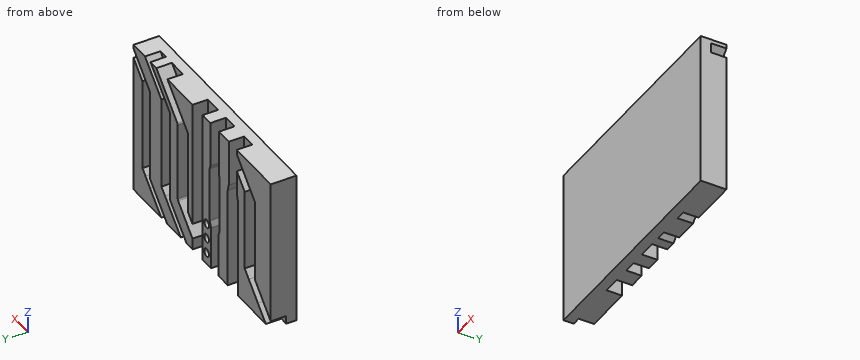
```python
from build123d import *

# Parameters (mm, degrees)
SKETCH1_W           = 292.1
SKETCH1_H           = 190.5
BOSS_EXTRUDE1_DEPTH = 31.75
CUT_EXTRUDE1_DEPTH  = 19.05
FILLET1_R           = 3.175
SKETCH8_R           = 5.08
CUT_EXTRUDE2_DEPTH  = 12.7
CUT_EXTRUDE3_DEPTH  = 19.05
CUT_EXTRUDE4_START  = -19.05
CUT_EXTRUDE4_DEPTH  = 19.05


with BuildPart() as part:
    # Sketch1 → Boss-Extrude1 (new body)
    with BuildSketch(Plane(origin=(0, 0, 0), x_dir=(1, 0, 0), z_dir=(0, 1, 0))):
        Rectangle(SKETCH1_W, SKETCH1_H)
    extrude(amount=BOSS_EXTRUDE1_DEPTH)

    # Sketch5 → Cut-Extrude1 (cut)
    with BuildSketch(Plane(origin=(0, 31.75, 0), x_dir=(1, 0, 0), z_dir=(0, 1, 0))):
        Polygon((-54.537973011, 56.645897063), (-54.537973011, 45.282587268), (-54.537973011, -9.143020761), (-54.537973011, -29.727810076), (-56.751368127, -37.988313106), (-56.751368127, -113.256317169), (-73.902361837, -113.256317169), (-73.902361837, -37.988313106), (-76.115756953, -29.727810076), (-76.115756953, -11.930912732), (-76.115756953, -9.143020761), (-76.115756953, 45.282587268), (-76.115756953, 56.645897063), (-76.115756953, 64.900897063), (-76.115756953, 123.938542293), (-54.537973011, 123.938542293), (-54.537973011, 64.900897063), align=None)
        Polygon((-35.869641097, -54.76875), (-35.869641097, -113.256317169), (-17.739641097, -113.256317169), (-17.739641097, -54.76875), (-17.739641097, -38.54651566), (-16.168929869, -34.231022029), (-16.168929869, 34.231022029), (-19.014641097, 42.04954937), (-19.014641097, 54.76875), (-19.014641097, 123.938542293), (-34.594641097, 123.938542293), (-34.594641097, 54.76875), (-34.594641097, 42.04954937), (-37.440352325, 34.231022029), (-37.440352325, -34.231022029), (-35.869641097, -38.54651566), align=None)
        Polygon((68.007088005, -12.827), (68.007088005, -53.93599914), (75.733185186, -61.662096321), (85.826970956, -71.755882091), (120.911645373, -106.060842413), (128.794129656, -102.532519884), (91.922231409, -65.660621637), (86.625610633, -60.36400086), (86.625610633, -12.827), (86.625610633, 12.827), (86.625610633, 54.107702226), (78.899513451, 61.662096321), (69.164333129, 71.397276643), (30.279619459, 110.281990313), (23.687738087, 104.683350778), (63.069072676, 65.302016189), (68.007088005, 60.36400086), (68.007088005, 12.827), align=None)
        Polygon((20.489996677, 80.981024842), (20.489996677, 107.787781329), (-1.087787265, 107.787781329), (-1.087787265, 37.36975), (-1.087787265, -17.055858029), (-1.087787265, -113.256317169), (20.489996677, -113.256317169), (20.489996677, -17.055858029), (20.489996677, 37.36975), (20.489996677, 61.776004665), (30.279619459, 51.986381883), (30.279619459, -51.734938461), (111.842171541, -133.297490543), (131.611931441, -129.619589579), (51.857403402, -49.865061539), (51.857403402, 49.613618117), align=None)
    extrude(amount=-CUT_EXTRUDE1_DEPTH, mode=Mode.SUBTRACT)

    # Fillet1
    fillet1_edges = [part.edges().sort_by_distance(p)[0] for p in [
        (-34.594641097, 22.225, -42.04954937),
        (-17.739641097, 22.225, 38.54651566),
        (-37.440352325, 22.225, 34.231022029),
        (-37.440352325, 22.225, -34.231022029),
        (-19.014641097, 22.225, -42.04954937),
        (-16.168929869, 22.225, -34.231022029),
        (-16.168929869, 22.225, 34.231022029),
        (-35.869641097, 22.225, 38.54651566),
        (51.857403402, 22.225, 49.865061539),
        (51.857403402, 22.225, -49.613618117),
        (30.279619459, 22.225, 51.734938461),
        (30.279619459, 22.225, -51.986381883),
        (-76.115756953, 22.225, 29.727810076),
        (-56.751368127, 22.225, 37.988313106),
        (-73.902361837, 22.225, 37.988313106),
        (-54.537973011, 22.225, 29.727810076),
    ]]
    fillet(fillet1_edges, radius=FILLET1_R)

    # Sketch8 → Cut-Extrude2 (cut)
    with BuildSketch(Plane(origin=(0, 31.75, 0), x_dir=(1, 0, 0), z_dir=(0, 1, 0))):
        with Locations(Location((-9.751260883, 42.41224903, 0), (0, 0, 270))):
            Circle(SKETCH8_R)
        with Locations(Location((-9.751260883, 61.46224903, 0), (0, 0, 270))):
            Circle(SKETCH8_R)
        with Locations(Location((-9.751260883, 80.51224903, 0), (0, 0, 270))):
            Circle(SKETCH8_R)
    extrude(amount=-CUT_EXTRUDE2_DEPTH, mode=Mode.SUBTRACT)

    # Sketch10 → Cut-Extrude3 (cut)
    with BuildSketch(Plane(origin=(0, 31.75, 0), x_dir=(1, 0, 0), z_dir=(0, 1, 0))):
        Polygon((110.861963616, 12.827), (110.861963616, -12.827), (110.861963616, -55.20599914), (117.318060797, -61.662096321), (127.591928077, -71.935963601), (167.375411749, -111.719447273), (167.375411749, -99.528926365), (133.687188531, -65.840703147), (126.940486244, -59.09400086), (126.940486244, -12.827), (126.940486244, 12.827), (126.940486244, 55.20599914), (120.484389062, 61.662096321), (110.927960718, 71.218524666), (71.315632765, 110.830852619), (59.125111857, 110.830852619), (104.832700264, 65.123264212), (110.861963616, 59.09400086), align=None)
    extrude(amount=-CUT_EXTRUDE3_DEPTH, mode=Mode.SUBTRACT)

    # Sketch13 → Cut-Extrude4 (cut)
    with BuildSketch(Plane(origin=(0, 31.75, 0), x_dir=(1, 0, 0), z_dir=(0, 1, 0)).offset(CUT_EXTRUDE4_START)):
        Polygon((-90.636160304, -19.2405), (-90.636160304, 19.2405), (-90.636160304, 50.320724899), (-99.345622638, 59.030187232), (-118.720884143, 78.405448738), (-162.613070171, 122.297634766), (-162.613070171, 101.678401026), (-129.030501013, 68.095831868), (-112.213944246, 51.279275101), (-112.213944246, 19.2405), (-112.213944246, -19.2405), (-112.213944246, -51.02783168), (-103.858035303, -59.383740623), (-84.482773798, -78.759002128), (-70.58319311, -92.658582816), (-70.58319311, -70.625135514), (-73.466050147, -67.742278477), (-90.636160304, -50.57216832), align=None)
    extrude(amount=CUT_EXTRUDE4_DEPTH, mode=Mode.SUBTRACT)


solid = part.part
```
The listing builds one solid part. Answer for the finished solid, in the listing's coordinates (mm). Give positions to 0.01 mm unless a question says otherwise; leave off trailing zeros. Write each loop counter-clockwise with the first axis right and the second up, starting at its lowest first coordinate (ties: lowest second). Pieces come first, ordered by that corner, then holes. Notation, with made-up numbers: (7.5, 36) -> (35.5, 36) arc R5 ccw to (35.5, 42) -> close; hole circle Ø8 at (51.25, -38). An arc over 180 degrees is marked (long way). Write item = value, one per line. Start each with the question number.
1) The part is cut by section A-A, the plane x = 105.5. Determine the outline of the cut face in (y, z).
2) Straight lines are drawn through the part: line 1 along Z through (x, y) = (62, 18.5); line 2 along Z through (x, y) = (66, 25); line 3 along Z through (x, y) = (34, 15.5). For each, find the intervals that lie inside material, in ascending order.
3) This flat-tipped pin is pushed along its axis until it touches: pin 1 (3 mm diameter, centred on x = -11.5, z = -62, fed in from +Y). Where does it stop, or does it pass through?
4) The part is cut by section B-B, the plane y = 28. Count the separate pieces of the cut face and the enclosed holes in it, and give its area (3 significant figures).
5) The part is cut by section C-C, the plane x = -31. Determine the outline of the cut face in (y, z).
Solutions:
q1.outline = (0, -95.25) -> (31.75, -95.25) -> (31.75, -76.65) -> (12.7, -76.65) -> (12.7, -64.46) -> (31.75, -64.46) -> (31.75, 79.24) -> (12.7, 79.24) -> (12.7, 90.99) -> (31.75, 90.99) -> (31.75, 95.25) -> (0, 95.25) -> close
q2.line_1 = -95.25 to -78.56, -66.37 to 60.01, 83.46 to 95.25
q2.line_2 = -95.25 to -74.56, -62.37 to 64.01, 87.46 to 95.25
q2.line_3 = -94.37 to -67.47, 55.46 to 95.25
q3.pin_1 = 19.05
q4.separate_pieces = 8
q4.enclosed_holes = 3
q4.area = 30,900 mm²
q5.outline = (0, -95.25) -> (12.7, -95.25) -> (12.7, 95.25) -> (0, 95.25) -> close
